Autodesk Inventor part; units mm, degrees
ref_plane "YZ Plane" through (0, 0, 0) normal (1, 0, 0) x (0, 1, 0)
ref_plane "XZ Plane" through (0, 0, 0) normal (0, 1, 0) x (-1, 0, 0)
ref_plane "XY Plane" through (0, 0, 0) normal (0, 0, 1) x (1, 0, 0)
sketch "Sketch1" plane through (0, 0, 0) normal (0, 0, 1) x (1, 0, 0)
  circle A0 centre (0, 0) radius 30.1
  circle A1 centre (0, 0) radius 31.9
  dimension "d0" = 60.2
  dimension "d1" = 63.8
extrude "Extrusion1" add sketch "Sketch1" along normal blind 5.8
sketch "Sketch2" plane through (0, 0, 5.8) normal (0, 0, 1) x (1, 0, 0)
  line L0 (-0.15, 30.6) -> (0.15, 30.6)
  line L1 (0.15, 30.6) -> (0.15, 28.6)
  line L2 (0.15, 28.6) -> (-0.15, 28.6)
  line L3 (-0.15, 28.6) -> (-0.15, 30.6)
  line L4 (-0.15, -33.5) -> (0.15, -33.5)
  line L5 (0.15, -33.5) -> (0.15, -31.5)
  line L6 (0.15, -31.5) -> (-0.15, -31.5)
  line L7 (-0.15, -31.5) -> (-0.15, -33.5)
  point P0 (0, 0)
  point P1 (0, 28.6)
  point P2 (0, -31.5)
  dimension "d7" = 30.6
  dimension "d8" = 0.3
  dimension "d9" = 2
  dimension "d10" = 31.5
  dimension "d11" = 2
extrude "Extrusion2" cut sketch "Sketch2" against normal through all
chamfer "Chamfer1" distance 0.4 angle 45 8 edges at (-22.5036, 22.6097, 5.8) (22.6097, -22.5036, 5.8) (21.3369, 21.2308, 5.8) (-21.2308, -21.3369, 5.8) (-22.5036, 22.6097, 0) (22.6097, -22.5036, 0) (21.3369, 21.2308, 0) (-21.2308, -21.3369, 0)
properties part number "light-seam" material "ABS Plastic"
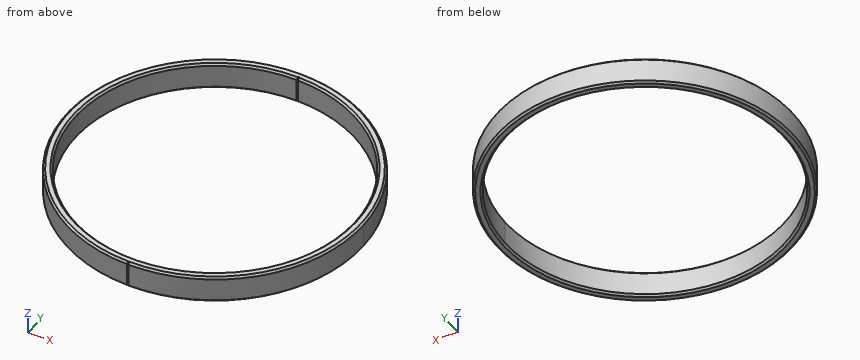
Could you check a few things on this model? Use its own coordinates, in mm. Give positions to 0.01 mm unless a question says otherwise; leave off trailing zeros. Write each loop counter-clockwise with the first axis right and the second up, starting at its lowest first coordinate (ties: lowest second). Pieces come first, ordered by that corner, then holes. Notation, with made-up numbers: (42, -36.75) -> (71, -36.75) arc R17 cw to (71, -23.75) -> close; hole circle Ø11 at (88.25, 0). An arc over 180 degrees is marked (long way). Write each question's results on one line, items separated by ' | '.
1. Will these pins go through, and if not, where does the flat tip stop? pin 1 Ø1.5 at (x, z) = (-6.5, 3.5) entering from +Y; pin 2 Ø2 at (x, z) = (24, 5) entering from -Y; pin 3 Ø1.5 at (x, z) = (-9.5, 2) entering from +Y; pin 4 Ø8 at (x, y) = (-13, -22) entering from +Z.
Check sheet entries:
pin 1: stops at y = 31.38 | pin 2: stops at y = -22.1 | pin 3: stops at y = 30.68 | pin 4: passes through
2. I want a section at A-A, the plane z = 3.35. Write out the boundary of the cut face in (x, y).
Check sheet entries:
outline: (-0.15, -31.9) -> (-0.15, -31.5) -> (0.15, -31.5) -> (0.15, -31.9) arc R31.9 ccw (long way) to start; hole (-0.15, 30.1) arc R30.1 ccw (long way) to (0.15, 30.1) -> (0.15, 30.6) -> (-0.15, 30.6) -> close
3. I need wall thicknesses on L1, parallel to Y at x = 0, z = 3.2; L2, parallel to X at y = 0, z = 3.9; L3, parallel to X at y = -6, z = 1.85. Which ranges of each line are inside material? Lowest first, please.
Check sheet entries:
L1: y = -31.5 to -30.1, 30.6 to 31.9 | L2: x = -31.9 to -30.1, 30.1 to 31.9 | L3: x = -31.33 to -29.5, 29.5 to 31.33
